The listing builds one solid part. Answer for the finished solid, in the listing's coordinates (mm). Face numbers are marked on the shaded views. Round coordinates to 2 decimals unless told otherwise and drop trailing zeros. Write each loop counter-clockwise with the first axis right and the second up, starting at its lowest first coordinate (ties: lowest second). Pieces come first, ordered by that corner, then holes. Notation, with made-up numbers: (85, 23.5) - (105, 23.5) arc R17 ccw to (105, 49.5) - close; hole circle Ø5 at (-18.75, 55). An arc over 180 degrees is marked (long way). Answer in a Markdown table with one row per item.
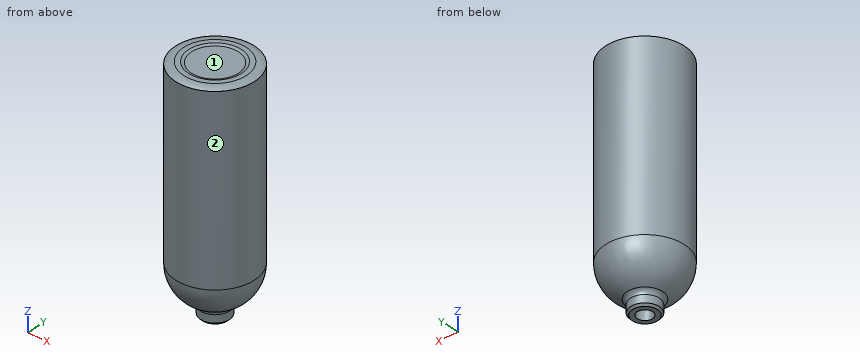
from build123d import *


with BuildPart() as part:
    # Sketch1 → Revolve1 (revolve)
    with BuildSketch(Plane(origin=(0, 0, 0), x_dir=(1, 0, 0), z_dir=(0, 1, 0))):
        with BuildLine():
            Line((-34, -46.163818636), (0, -46.163818636))
            Line((0, -46.163818636), (0, -52.268618281))
            Line((0, -52.268618281), (-24.5, -52.268618281))
            Line((-24.5, -52.268618281), (-27.5, -53.268618281))
            Line((-27.5, -53.268618281), (-32.5, -53.268618281))
            ThreePointArc((-32.5, -53.268618281), (-36.885372769, -52.719543337), (-41, -51.106217468))
            Line((-41, -51.106217468), (-41, 136.731381719))
            ThreePointArc((-41, 136.731381719), (-34.81270119, 157.603387492), (-18.25, 171.731381719))
            ThreePointArc((-18.25, 171.731381719), (-15.88389983, 173.749666608), (-15, 176.731381719))
            Line((-15, 176.731381719), (-15, 184.731381719))
            Line((-15, 184.731381719), (-13, 186.731381719))
            Line((-13, 186.731381719), (-8, 186.731381719))
            Line((-8, 186.731381719), (-8, 179.731381719))
            Line((-8, 179.731381719), (-8, 176.731381719))
            ThreePointArc((-8, 176.731381719), (-10.014794516, 169.934748154), (-15.408172232, 165.33419367))
            ThreePointArc((-15.408172232, 165.33419367), (-28.943595876, 153.788469038), (-34, 136.731381719))
            Line((-34, 136.731381719), (-34, -46.163818636))
        make_face()
    revolve(axis=Axis((0, 0, 52.268618281), (0, 0, -1)))


solid = part.part
(1) Section A-A (z = -3.5) is taken. Give the vertices of the cut face in (x, y), and give its area (3 significant figures).
Checked values:
| item | result |
|---|---|
| outline | circle Ø82 at (0, 0); hole circle Ø68 at (0, 0) |
| area | 1,650 mm2 |
(2) For a pull along X with two mould halves and no side action, classify the marked faces 1 and 2 as pulls with the +X half, pulls with the -X half, needs draft (parallel to the pull), parting line crosses it, or undercut.
Checked values:
| item | result |
|---|---|
| face 1 | undercut |
| face 2 | parting line crosses it |
(3) Flat-ended cylindrical pins translate along their axes: pin 1 (12 mm diameter, centred on x = 31, y = 30, fed in from -Z); pin 2 (12 mm diameter, centred on x = 13, z = -42, fed in from -Y); pin 3 (2 mm diameter, centred on x = -5.5, y = 32.5, fed in from -Z). Find the tip coordinate at first contact, or state that the pin passes through.
Checked values:
| item | result |
|---|---|
| pin 1 | stops at z = -153.49 |
| pin 2 | stops at y = -40.4 |
| pin 3 | stops at z = -161.44 |
(4) Find the intervals of material crossed by line 1 (Y direction, x = 0, z = -29.5); line 2 (Y direction, x = 0, z = -184.25); line 3 (X direction, y = 25, z = -85.5), in increasing order.
Checked values:
| item | result |
|---|---|
| line 1 | y = -41 to -34, 34 to 41 |
| line 2 | y = -15 to -8, 8 to 15 |
| line 3 | x = -32.5 to -23.04, 23.04 to 32.5 |
